from build123d import *

# Parameters (mm, degrees)
F0_R          = 4.7625
F1_DEPTH      = 25.4
F2_W          = 6.35
F2_H          = 4.7452268491
F5_DEPTH      = 4.7635
F5_DEPTH_BACK = 4.7635
F6_R          = 2.38125
F7_DEPTH      = 12.7


with BuildPart() as f1:
    # F0 (on Front) → F1 (new body)
    with BuildSketch(Plane.XZ):
        Circle(F0_R)
    extrude(amount=F1_DEPTH)

    # F2 (on Right) → F3 (revolve, cut)
    with BuildSketch(Plane.YZ):
        with Locations((-22.225, 4.7500534246)):
            Rectangle(F2_W, F2_H)
    revolve(axis=Axis((0, -25.3480933607, 0), (0, -1, 0)), mode=Mode.SUBTRACT)

    # F4 (on Right) → F5 (cut, two sides)
    with BuildSketch(Plane.YZ) as f5_sk:
        Polygon((0, -1.5875), (0, 0), (0, 1.5875), (-12.7, 1.5875), (-12.7, 0), (-12.7, -1.5875), align=None)
    extrude(amount=-F5_DEPTH, mode=Mode.SUBTRACT)
    extrude(f5_sk.sketch, amount=F5_DEPTH_BACK, mode=Mode.SUBTRACT)

    # F6 (on Top) → F7 (cut, symmetric)
    with BuildSketch(Plane.XY):
        with Locations((0, -3.81)):
            Circle(F6_R)
    extrude(amount=F7_DEPTH, both=True, mode=Mode.SUBTRACT)


solid = f1.part
The model under review builds one solid part; all positions refer to its coordinate system, in mm. A direction names the side the tool comes from. Coordinates: 2 decimals unless noted, no trailing zeros. Loops run counter-clockwise (first coordinate to the right, second up) from the corner with the lowest first, then second, coordinate; pieces in that order, holes last. Notation, with made-up numbers: M -35,72.25 L 11,72.25 A13 cw 11,84.25 Z; hole C 39,41 d11. An arc over 180 degrees is marked long. Put each result on its own line as item: value. Start each with the question number.
Q1. Add section D-D (y = -11). Write out the cut boundary in (x, z) (1 decimal), and give its area (3 significant figures).
Q2. Clearance check with flat-ended pins moving along their axes: pin 1 (3 mm diameter, centred on y = -14, z = -3.5, fed in from +X); pin 2 (2 mm diameter, centred on x = -1.5, y = -3, fed in from +Z); pin 3 (4 mm diameter, centred on x = -2, y = -17.5, fed in from -Z); pin 4 (1.6 mm diameter, centred on x = -2, z = 0, fed in from +Y). State where each tip first meets the part, or that it passes through.
Q3. Add section A-A (x = 0). Write out the cut boundary in (y, z).
Q4. Wall thickness on line 1 (Y direction, x = 0, z = -4.05); line 2 (Y direction, x = -3.25, z = 1); line 3 (Y direction, x = -1.5, z = 3.25): over which ranges is each line inside the solid? List them lowest first.
Q5. Add section C-C (z = 2). Write out the cut boundary in (x, y), and give its area (3 significant figures).
Q6. The part is to be moulded in two halves that separate along Z. For faces 4 (the flat face through (0.1, -6.4, -1.588)), 5 (the flat face through (2, -19.05, -2)), 6 (the cylindrical face through (2.198, -9.392, -4.225)), say which applies: +Z half, -Z half, draft (parallel to the pull), parting line (faces both ways), or undercut.
Q7. For faces 1 (the flat face through (0, 0, -3)), 2 (the flat face through (0, -12.7, 0)), 3 (the cylindrical face through (-0.71, -22.18, 2.27)), list the 3-axis set-ups (+Z, -Z, +X, -X, +Y, -Y) from which the entire face can be reached by the end or side of a thin tool; tool diameter is ignored.
Q8. Add section B-B (y = -5.25). Write out the cut boundary in (x, z) (1 decimal).
Answers:
1. outline: M -4.5,-1.6 A4.8 ccw 4.5,-1.6 Z; M -4.5,1.6 L 4.5,1.6 A4.8 ccw Z
1. area: 41.6 mm^2
2. pin 1: stops at x = 4.32
2. pin 2: stops at z = 4.5
2. pin 3: stops at z = -4.76
2. pin 4: stops at y = -12.7
3. outline: M -25.4,-2.38 L -19.05,-2.38 L -19.05,-4.76 L -6.19,-4.76 L -6.19,-1.59 L -12.7,-1.59 L -12.7,1.59 L -6.19,1.59 L -6.19,4.76 L -19.05,4.76 L -19.05,2.38 L -25.4,2.38 Z; M -1.43,-4.76 L 0,-4.76 L 0,-1.59 L -1.43,-1.59 Z; M -1.43,1.59 L 0,1.59 L 0,4.76 L -1.43,4.76 Z
4. line 1: y = -19.05 to -6.19, -1.43 to 0
4. line 2: y = -19.05 to -12.7
4. line 3: y = -19.05 to -5.66, -1.96 to 0
5. outline: M -4.32,-19.05 L -1.29,-19.05 L -1.29,-25.4 L 1.29,-25.4 L 1.29,-19.05 L 4.32,-19.05 L 4.32,0 L -4.32,0 Z; hole C 0,-3.81 d4.76
5. area: 163 mm^2
6. face 4: undercut
6. face 5: draft
6. face 6: parting line
7. face 1: +Z, -Z, +X, -X, +Y
7. face 2: +X, -X, +Y
7. face 3: -Y
8. outline: M -4.5,-1.6 A4.8 ccw -1.9,-4.4 L -1.9,-1.6 Z; M -4.5,1.6 L -1.9,1.6 L -1.9,4.4 A4.8 ccw Z; M 1.9,-4.4 A4.8 ccw 4.5,-1.6 L 1.9,-1.6 Z; M 1.9,1.6 L 4.5,1.6 A4.8 ccw 1.9,4.4 Z
